Autodesk Inventor part; units mm, degrees
ref_plane "YZ Plane" through (0, 0, 0) normal (1, 0, 0) x (0, 1, 0)
ref_plane "XZ Plane" through (0, 0, 0) normal (0, 1, 0) x (-1, 0, 0)
ref_plane "XY Plane" through (0, 0, 0) normal (0, 0, 1) x (1, 0, 0)
sketch "Skizze1" plane through (0, 0, 0) normal (0, 0, 1) x (1, 0, 0)
  line L0 (0, 0) -> (-2, 0)
  line L1 (-2, 0) -> (-2, -1)
  line L2 (-2, -1) -> (-3, -1)
  line L3 (-3, -1) -> (-3, 9)
  line L4 (-3, 9) -> (-2, 9)
  line L5 (-2, 9) -> (-2, 8)
  line L6 (-2, 8) -> (0, 8)
  line L7 (0, 8) -> (0, 0)
  line L8 (10.5, 10.652115) -> (10.5, -3.008314) construction
  dimension "d0" = 3
  dimension "d1" = 10
  dimension "d2" = 8
  dimension "d3" = 1
  dimension "d4" = 2
  dimension "d5" = 10.5
sketch "Skizze1 outline for Umdrehung1" plane through (0, 0, 0) normal (0, 0, 1) x (1, 0, 0)
  line L0 (0, 0) -> (-2, 0)
  line L1 (-2, 0) -> (-2, -1)
  line L2 (-2, -1) -> (-3, -1)
  line L3 (-3, -1) -> (-3, 9)
  line L4 (-3, 9) -> (-2, 9)
  line L5 (-2, 9) -> (-2, 8)
  line L6 (-2, 8) -> (0, 8)
  line L7 (0, 8) -> (0, 0)
revolve "Umdrehung1" add sketch "Skizze1 outline for Umdrehung1" angle 360 about axis through (10.5, 10.652115, 0) along (0, -1, 0)
sketch "Skizze2" plane through (10.5, -1, 0) normal (0, -1, 0) x (1, 0, 0)
  circle A0 centre (0, 0) radius 13.5 construction
  line L0 (-13.499999, -0.004969) -> (1.488599, -0.004969) construction
  line L1 (-13.5, 14.995031) -> (-27.5, 14.995031)
  line L2 (-27.5, 14.995031) -> (-27.5, 9.995031)
  circle A1 centre (0, 0) radius 12.5 construction
  circle A2 centre (0, 0) radius 13.5
  circle A3 centre (0, 0) radius 12.5
  circle A4 centre (0, 0) radius 12.5
  line L3 (-27.5, 9.995031) -> (-14.5, 9.995031)
  line L4 (-14.5, 9.995031) -> (-13.499999, -0.004969)
  line L5 (-0.042524, -33.95519) -> (-0.042524, 19.973998) construction
  line L6 (13.414952, 14.995031) -> (27.414952, 14.995031)
  line L7 (27.414952, 14.995031) -> (27.414952, 9.995031)
  line L8 (12.499991, -0.004969) -> (13.414952, 14.995031)
  line L9 (27.414952, 9.995031) -> (14.414952, 9.995031)
  line L10 (14.414952, 9.995031) -> (13.414951, -0.004969)
  line L11 (-13.5, 14.995031) -> (-12.499999, -0.004969)
  circle A5 centre (0, 0) radius 12.5
  line L12 (-12.499999, -0.004969) -> (-13.499999, -0.004969)
  line L13 (13.414951, -0.004969) -> (12.499991, -0.004969)
  point P0 (-10.5, 0)
  point P1 (10.414952, 0)
  dimension "d9" = 15
  dimension "d11" = 5
  dimension "d12" = 13
  dimension "d13" = 14
  dimension "d14" = 27.5
sketch "Skizze2 outline for Extrusion1" plane through (10.5, -1, 0) normal (0, -1, 0) x (1, 0, 0)
  line L0 (12.499991, -0.004969) -> (13.414951, -0.004969)
  line L1 (13.414952, 14.995031) -> (12.499991, -0.004969)
  line L2 (27.414952, 14.995031) -> (13.414952, 14.995031)
  line L3 (27.414952, 9.995031) -> (27.414952, 14.995031)
  line L4 (14.414952, 9.995031) -> (27.414952, 9.995031)
  line L5 (13.414951, -0.004969) -> (14.414952, 9.995031)
  line L6 (-13.499999, -0.004969) -> (-14.5, 9.995031)
  line L7 (-14.5, 9.995031) -> (-27.5, 9.995031)
  line L8 (-27.5, 9.995031) -> (-27.5, 14.995031)
  line L9 (-27.5, 14.995031) -> (-13.5, 14.995031)
  line L10 (-13.5, 14.995031) -> (-12.499999, -0.004969)
  line L11 (-12.499999, -0.004969) -> (-13.499999, -0.004969)
extrude "Extrusion1" add sketch "Skizze2 outline for Extrusion1" against normal blind 11.5 and the other way blind 1.5
sketch "Skizze5" plane through (-17, -2.5, 14.995031) normal (-1, 0, 0) x (0, 0, 1)
  line L0 (-15, 13) -> (-15, 11.5)
  line L1 (-5, 13) -> (-5, 0)
  line L2 (-15, 11.5) -> (-5, 13)
  line L3 (-5, 13) -> (-15, 13)
  line L4 (-15, 13) -> (-15, 11.5)
  line L5 (-15, 1.5) -> (-15, 11.5)
  line L6 (-15, 1.5) -> (-5, 0)
  line L7 (0, 0) -> (-15, 0)
  line L8 (-15, 1.5) -> (-15, 0)
  line L9 (-15, 0) -> (-15, 1.5)
  line L10 (-15, 0) -> (-5, 0)
  point P0 (-14.995031, 2.5)
sketch "Skizze5 outline for Extrusion4" plane through (-17, -2.5, 14.995031) normal (-1, 0, 0) x (0, 0, 1)
  line L0 (-15, 13) -> (-15, 11.5)
  line L1 (-5, 13) -> (-15, 13)
  line L2 (-15, 11.5) -> (-5, 13)
  line L3 (-5, 0) -> (-15, 1.5)
  line L4 (-15, 0) -> (-5, 0)
  line L5 (-15, 1.5) -> (-15, 0)
extrude "Extrusion4" cut sketch "Skizze5 outline for Extrusion4" against normal through all
chamfer "Fase1" distance 2 angle 45 4 edges at (-17, -2.5, 12.495) (-17, 10.5, 12.495) (37.915, -2.5, 12.495) (37.915, 10.5, 12.495)
hole "Bohrung1" at (31.414952, 4, 9.995031) direction (0, 0, 1) diameter 4.5 end through all
hole "Bohrung2" at (-10.5, 4, 9.995031) direction (0, 0, 1) diameter 4.5 end through all
properties part number "lagerblock" material "Gusseisen, grau, ASTM A48 Klasse 20"
CAD build for the part. Positions are in the model's coordinates, mm. A direction names the side the tool comes from. Round coordinates to 2 decimals unless told otherwise and drop trailing zeros. Write each loop counter-clockwise with the first axis right and the second up, starting at its lowest first coordinate (ties: lowest second). Pieces come first, ordered by that corner, then holes. Notation, with made-up numbers: (-19, 51) - (38, 51) arc R13 ccw to (38, 67) - close; hole circle Ø9 at (12, 81). An arc over 180 degrees is marked (long way). Return JSON: item names as keys, results as strings. Group by question number.
Item 1: Probe probe 1 along Y at (x, z) = (-10.5, 13.4); probe 2 along X at (y, z) = (7, 8.75); probe 3 along Z at (x, y) = (10.5, 8.7). List the from-to ranges inside material, lowest first.
Item 2: Band-saw the part on B-B on y = 4. List the corners of the cut face in (x, z).
Item 3: Band-saw the part on C-C on z = 1.5. List the corners of the cut face in (x, y), plus the area to 3 significant figures.
Item 4: 3-axis set-ups, long thin cutter, end or side, ignore diameter. For faces 4 (the face through (11, 9, -13)), 5 (the face through (23.94, -1.76, 5.07)), 6 (the face through (19.71, 8.49, -8.45)): which of +Z, -Z, +X, -X, +Y, -Y reach the whole face in a straight line?
Item 5: Band-saw the part on A-A on x = -10.5. List the corners of the cut face in (y, z), plus the area to 3 significant figures.
Item 6: Band-saw the part on D-D on x = 10.5. List the corners of the cut face in (y, z), plus the area to 3 significant figures.
Item 7: Mould opens along X. For faces 1 (the face through (-16, -1.5, 12.5)), 2 (the face through (28, 4, 9.995)), 3 (the face through (0.5, 3.9, -3.2)) say: +X half, -X half, draft (parallel to the pull), parting line (faces both ways), or undercut.
Item 8: Flat gauge pins, fed straight in: pin 1 Ø4 at (y, z) = (-1, -7.5) entering from -X; pin 2 Ø1.5 at (y, z) = (0.5, 4) entering from -X; pin 3 Ø5 at (x, y) = (-11, 0) entering from -Z; pin 4 Ø3.5 at (x, y) = (-10.5, 4) entering from +Z (3 decimals). Where does each tip first touch, or does it go through?
Resolved:
{
 "1": {"probe 1": "y = -2.5 to 1.75, 6.25 to 10.5", "probe 2": "x = -3.88 to -2.58, 0.22 to 4.7, 16.3 to 20.78, 23.53 to 24.79", "probe 3": "z = -13.5 to -12.5, 12.5 to 13.5"},
 "2": {"outline": "(-17, 10) - (-12.75, 10) - (-12.75, 15) - (-17, 15) - close; (-8.25, 10) - (-4, 10) - (-3, 0) arc R13.5 ccw (long way) to (23.98, 0.68) - (24.91, 10) - (29.16, 10) - (29.16, 15) - (23.91, 15) - (23.27, 4.39) arc R13.5 ccw to (-2.29, 4.32) - (-3, 15) - (-8.25, 15) - close; (33.66, 10) - (37.91, 10) - (37.91, 15) - (33.66, 15) - close; hole circle Ø21 at (10.5, 0)"},
 "3": {"outline": "(-3.15, -1.23) - (-2.1, -1.23) - (-2.1, -1) - (-1.91, -1) - (-1.91, 0) - (0.11, 0) - (0.11, 8) - (-1.91, 8) - (-1.91, 9) - (-2.1, 9) - (-2.1, 9.23) - (-3.15, 9.23) - close; (20.89, 0) - (22.91, 0) - (22.91, -1) - (23.09, -1) - (23.09, -1.23) - (24.07, -1.23) - (24.07, 9.23) - (23.09, 9.23) - (23.09, 9) - (22.91, 9) - (22.91, 8) - (20.89, 8) - close", "area": "57.2 mm²"},
 "4": {"face 4": "-Z, +X, -X, +Y", "face 5": "-Z, +X, -X, -Y", "face 6": "+Y"},
 "5": {"outline": "(-2.5, 10) - (1.75, 10) - (1.75, 15) - (-2.5, 15) - close; (6.25, 10) - (10.5, 10) - (10.5, 15) - (6.25, 15) - close", "area": "42.5 mm²"},
 "6": {"outline": "(-1, -13.5) - (9, -13.5) - (9, -12.5) - (8, -12.5) - (8, -10.5) - (0, -10.5) - (0, -12.5) - (-1, -12.5) - close; (-1, 12.5) - (0, 12.5) - (0, 10.5) - (8, 10.5) - (8, 12.5) - (9, 12.5) - (9, 13.5) - (-1, 13.5) - close", "area": "52.0 mm²"},
 "7": {"face 1": "-X half", "face 2": "draft", "face 3": "undercut"},
 "8": {"pin 1": "stops at x = -1.83", "pin 2": "stops at x = -3.48", "pin 3": "stops at z = 10", "pin 4": "passes through"}
}
